Design review of the part built by this model. Coordinates are the model's own, in mm. Round coordinates to 2 decimals unless told otherwise and drop trailing zeros. Order: outer loops, then holes, each group sorted by start corner. A loop starts at its lowest first (then second) coordinate and runs counter-clockwise, first axis right, second up. Notation, with made-up numbers: M 47.5,-14.75 L 56.5,-14.75 A15 cw 56.5,-6.75 Z; hole C 26.25,27.25 d5. An arc over 180 degrees is marked long. Use a Markdown table: item, result. Add a question column.
(1) To check wall thickness, follow probe 1 along X at (y, z) = (-7.5, 32); probe 2 along Y at (x, z) = (-8.75, 7.5); probe 3 along Y at (x, z) = (-8, 22.5). State the ranges of each line that lie inside material, in increasing order. Write a range as from..to.
(2) For pin 1 (6 mm diameter, centred on x = -6.5, y = -3, fed in from -Z); pin 2 (4 mm diameter, centred on x = -8.5, z = 11, fed in from +Y); pin 3 (8 mm diameter, centred on x = -7, y = -6.5, fed in from -Z), all flat-tipped, find the tip position at first contact; note any pin that passes through.
(3) Take a section at A-A (y = -16.5). Write out the cut boundary in (x, z).
(4) Take a section at B-B (x = -17.75). Write out the cut boundary in (y, z), then the cut area to 3 significant figures.
```python
from build123d import *

# Parameters (mm, degrees)
F0_W     = 19.5
F0_H     = 19.5
F0_W_2   = 6.6
F0_H_2   = 7.6
F1_DEPTH = 45
F3_DEPTH = 25
F4_W     = 6.6
F4_H     = 7.6
F5_DEPTH = 50
F5_TAPER = -0.3
F6_R     = 2


with BuildPart() as f1:
    # F0 (on Top) → F1 (new body)
    with BuildSketch(Plane.XY):
        with Locations((-9.75, -9.75)):
            Rectangle(F0_W, F0_H)
        with Locations((-9.75, -9.75)):
            Rectangle(F0_W_2, F0_H_2, mode=Mode.SUBTRACT)
    extrude(amount=F1_DEPTH)

    # F2 (on face) → F3 (cut)
    with BuildSketch(Plane.YZ):
        Polygon((0, 19.5), (-19.5, 0), (0, 0), align=None)
    extrude(amount=-F3_DEPTH, mode=Mode.SUBTRACT)

    # F4 (on Top) → F5 (cut)
    with BuildSketch(Plane.XY):
        with Locations((-9.75, -9.75)):
            Rectangle(F4_W, F4_H)
    extrude(amount=F5_DEPTH, taper=F5_TAPER, mode=Mode.SUBTRACT)

    # F6
    f6_edges = [f1.edges().sort_by_distance(p)[0] for p in [
        (-9.75, -5.714378, 45),
        (-13.285622, -9.75, 45),
        (-6.214378, -9.75, 45),
        (-9.75, -13.785622, 45),
    ]]
    fillet(f6_edges, radius=F6_R)


solid = f1.part
```
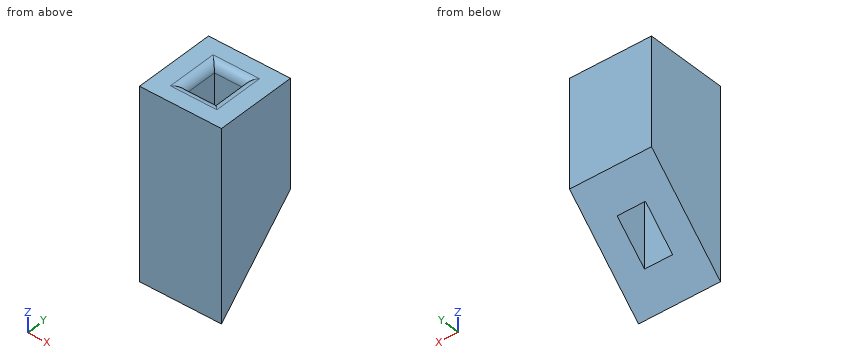
Verdict:
| question | item | result |
|---|---|---|
| 1 | probe 1 | x = -19.5..-13.22, -6.28..0 |
| 1 | probe 2 | y = -19.5..-13.59 |
| 1 | probe 3 | y = -19.5..-13.67, -5.83..0 |
| 2 | pin 1 | stops at z = 13.5 |
| 2 | pin 2 | stops at y = -13.6 |
| 2 | pin 3 | stops at z = 9.04 |
| 3 | outline | M -19.5,3 L 0,3 L 0,45 L -19.5,45 Z |
| 4 | outline | M -19.5,0 L 0,19.5 L 0,45 L -19.5,45 Z |
| 4 | area | 687 mm^2 |
